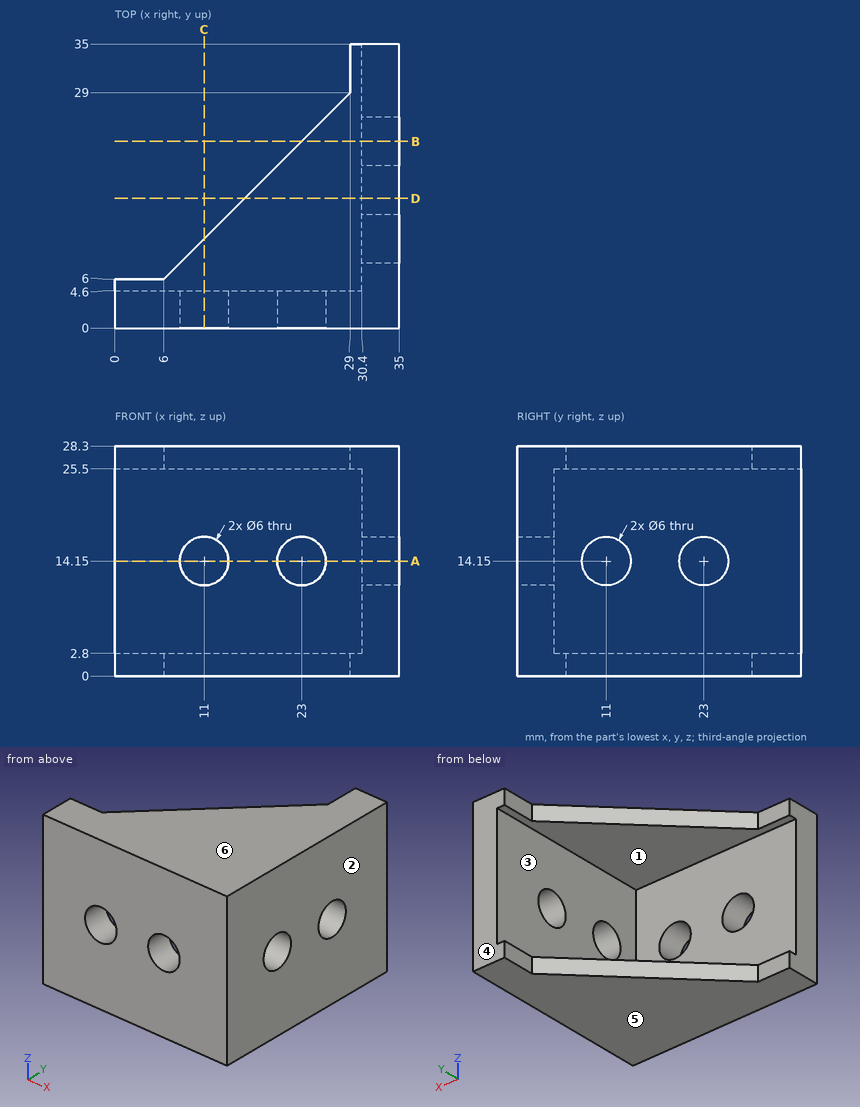
Answer from the drawing. Dimensions are ordinates in mm from the lowest x, y and z of the part. A direction names the side the tool comes from. Give positions to 0.01 mm unless a question says otherwise; leave off trailing zeros. Write each loop counter-clockwise with the first axis right and the second up, starting at its lowest first coordinate (ties: lowest second). Pieces come first, ordered by that corner, then holes. Notation, with made-up numbers: (21.5, 72.25) - (57.5, 72.25) arc R32 cw to (57.5, 102.25) - close; hole circle Ø3 at (-20.75, 86.5). An arc over 180 degrees is marked (long way). Answer in a Markdown table with one row per item. Add a question column.
Item 1: Section D-D, the plane y = 16 is taken. Write down the section's boundary in (x, z), and give its area (3 significant figures).
Item 2: Section B-B, the plane y = 23 is taken. Write down the section's boundary in (x, z).
Item 3: Find the intervals of material crossed by L1, parallel to Z at x = 11, y = 1.9; L2, parallel to X at y = 2.75, z = 14.15; L3, parallel to Z at x = 19.5, y = 7.5, in increasing order.
Item 4: Determine the mould class of the marked faces 3, 4, 5 and 6 for opening direction Z: pulls with the +Z half, pulls with the -Z half, needs draft (parallel to the pull), parting line crosses it, or undercut.
Item 5: Section C-C, the plane x = 11 is taken. Write down the section's boundary in (y, z).
Item 6: Flat-ended cylindrical pins translate along their axes: P1, Ø2, axis at y = 7.5, z = 5, coming from the -X side; P2, Ø10, axis at x = 6, z = 15.5, coming from the +Y side; P3, Ø0.8, axis at y = 30.5, z = 26.5, coming from the -X side. Find the tip coordinate at first contact, or state that the pin passes through.
Item 7: A tool of negligible diameter and unlimited length cuts with its end or side. For the marked faces 1 and 2, from which of +Z, -Z, +X, -X, +Y, -Y can it reach the whole face along a straight path? Write none if from no direction.
Item 8: Section A-A, the plane z = 14.15 is taken. Write down the section's boundary in (x, y).
Recorded:
| question | item | result |
|---|---|---|
| 1 | outline | (16, 0) - (35, 0) - (35, 28.3) - (16, 28.3) - (16, 25.5) - (30.4, 25.5) - (30.4, 2.8) - (16, 2.8) - close |
| 1 | area | 211 mm2 |
| 2 | outline | (23, 0) - (35, 0) - (35, 11.15) - (30.4, 11.15) - (30.4, 2.8) - (23, 2.8) - close; (23, 25.5) - (30.4, 25.5) - (30.4, 17.15) - (35, 17.15) - (35, 28.3) - (23, 28.3) - close |
| 3 | L1 | z = 0 to 11.15, 17.15 to 28.3 |
| 3 | L2 | x = 0 to 8, 14 to 20, 26 to 35 |
| 3 | L3 | z = 0 to 2.8, 25.5 to 28.3 |
| 4 | face 3 | undercut |
| 4 | face 4 | needs draft |
| 4 | face 5 | pulls with the -Z half |
| 4 | face 6 | pulls with the +Z half |
| 5 | outline | (0, 0) - (11, 0) - (11, 2.8) - (4.6, 2.8) - (4.6, 11.15) - (0, 11.15) - close; (0, 17.15) - (4.6, 17.15) - (4.6, 25.5) - (11, 25.5) - (11, 28.3) - (0, 28.3) - close |
| 6 | P1 | stops at x = 30.4 |
| 6 | P2 | stops at y = 4.6 |
| 6 | P3 | stops at x = 29 |
| 7 | face 1 | -X, +Y |
| 7 | face 2 | +Z, -Z, +X, +Y, -Y |
| 8 | outline | (0, 0) - (8, 0) - (8, 4.6) - (0, 4.6) - close; (14, 0) - (20, 0) - (20, 4.6) - (14, 4.6) - close; (26, 0) - (35, 0) - (35, 8) - (30.4, 8) - (30.4, 4.6) - (26, 4.6) - close; (30.4, 14) - (35, 14) - (35, 20) - (30.4, 20) - close; (30.4, 26) - (35, 26) - (35, 35) - (30.4, 35) - close |
